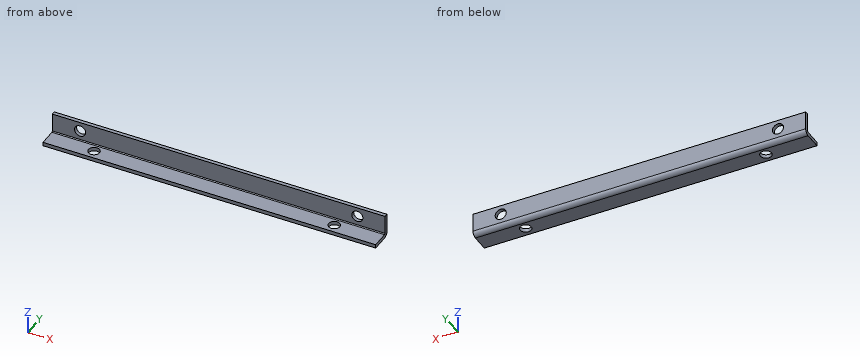
Autodesk Inventor part; units mm, degrees
ref_plane "YZ Plane" through (0, 0, 0) normal (1, 0, 0) x (0, 1, 0)
ref_plane "XZ Plane" through (0, 0, 0) normal (0, 1, 0) x (-1, 0, 0)
ref_plane "XY Plane" through (0, 0, 0) normal (0, 0, 1) x (1, 0, 0)
sketch "Boceto5" plane through (0, 0, 0) normal (0, 1, 0) x (-1, 0, 0)
  line L0 (10.2966, 28.3637) -> (10.2966, 8.3637)
  line L1 (10.2966, 8.3637) -> (-169.7034, 8.3637)
  line L2 (-169.7034, 8.3637) -> (-169.7034, 28.3637)
  line L3 (-169.7034, 28.3637) -> (10.2966, 28.3637)
  line L4 (10.2966, 18.3637) -> (-169.7034, 18.3637)
  circle A0 centre (-154.7034, 23.3637) radius 3
  circle A1 centre (-4.7034, 23.3637) radius 3
  circle A2 centre (-14.7034, 13.3637) radius 3
  circle A3 centre (-144.7034, 13.3637) radius 3
  point P0 (0, 0)
  dimension "d33" = 20
  dimension "d34" = 180
  dimension "d35" = 20
  dimension "d36" = 6
  dimension "d37" = 6
  dimension "d38" = 6
  dimension "d39" = 6
  dimension "d40" = 150
  dimension "d41" = 130
  dimension "d42" = 15
  dimension "d43" = 25
  dimension "d44" = 5
  dimension "d45" = 5
  dimension "d46" = 5
  dimension "d47" = 5
extrude "Extrusión4" add sketch "Boceto5" along normal blind 2 contours L0 L1 L2 L4
extrude "Extrusión5" add sketch "Boceto5" along normal blind 2 contours L0 L4 L2 L3
bend part "Pieza de plegado1" radius 0.5 angle 90 line through (-10.2966, 0, 18.3637) along (1, 0, 0) centre toward (0, -1, 0) moving side (0, 0, -1) both sides no
equation "\"Radio_pliegue\" = Grosor"
equation "\"Anchura_desahogo_plegado\" = Grosor"
equation "\"Profundidad_desahogo_plegado\" = 0.5 * Grosor"
equation "\"Tamaño_destalonado\" = 4 * Grosor"
equation "\"Remanente_mínimo\" = 2 * Grosor"
equation "\"Radiodetransición\" = Radio_pliegue"
equation "\"Tamaño_de_radio_de_Jacobi\" = Grosor"
equation "\"TamañoSeparación\" = Grosor"
properties part number "Soporte L" material "Aluminum 1100-H14"
Here's how the part is built. I have some questions about the finished solid (model axes, mm). Give positions to 0.01 mm unless a question says otherwise; leave off trailing zeros. Write each loop counter-clockwise with the first axis right and the second up, starting at its lowest first coordinate (ties: lowest second). Pieces come first, ordered by that corner, then holes. Notation, with made-up numbers: (73.5, -13) -> (131.5, -13) arc R15 cw to (131.5, -2) -> close; hole circle Ø4 at (9, 82.5). An arc over 180 degrees is marked (long way). Use one line per item in the form item = value.
1) I'm going to push flat-ended pins straight in: pin 1 (1.5 mm diameter, centred on y = -1, z = 18.5, fed in from -X); pin 2 (3.5 mm diameter, centred on x = 4.7, z = 23.36, fed in from -Y); pin 3 (5 mm diameter, centred on x = 40, z = 22.5, fed in from -Y). Where does each tip first touch, or does it pass through?
Verdict:
pin_1 = -10.3
pin_2 = through
pin_3 = 0
2) If I drill on L1, parallel to X at y = 1, z = 25.5; L2, parallel to Z at x = 104, y = -5.75; L3, parallel to Y at x = 26.5, z = 24.25, over which ranges is the centre line in solid material (lowest first)? Write a range as [from, to].
Verdict:
L1 = [-10.3, 2.6], [6.81, 152.6], [156.81, 169.7]
L2 = [15.86, 17.86]
L3 = [0, 2]
3) Suppose I cut it at A-A (x = 106). Please give me the cut outline in (y, z), and give its area (3 significant figures).
Verdict:
outline = (-9.71, 15.86) -> (-0.5, 15.86) arc R2.5 ccw to (2, 18.36) -> (2, 28.36) -> (0, 28.36) -> (0, 18.36) arc R0.5 cw to (-0.5, 17.86) -> (-9.71, 17.86) -> close
area = 43.1 mm2
